Can you work these out from the model? Positions are in its coordinate system, mm. A direction names the side the tool comes from. Coordinates: 2 decimals unless noted, no trailing zeros. Order: outer loops, then holes, each group sorted by start corner. A loop starts at its lowest first (then second) coordinate and runs counter-clockwise, first axis right, second up. Notation, with made-up numbers: (66, 75.5) -> (91, 75.5) arc R8 ccw to (91, 83.5) -> close; hole circle Ø11 at (70.5, 45.25). An arc over 180 degrees is marked (long way). Answer in a Markdown table with one row per item. Add a question column.
1. Will these pins go through, and if not, where does the flat tip stop? pin 1 (0.9 mm diameter, centred on x = -39, z = -1, fed in from +Y); pin 2 (3 mm diameter, centred on y = -1, z = 6.5, fed in from +X); pin 3 (8 mm diameter, centred on x = -14.5, y = 0, fed in from +Z).
2. Imagine slicing it at B-B on x = 14. Write out the boundary of the cut face in (y, z), plus the area to 3 significant figures.
3. On a 3-axis mill with a long thin cutter (end or side, diameter ignored), from which of +Z, -Z, +X, -X, +Y, -Y can I reach the whole of each face in a straight line? I mean faces 5 (the face through (-0.7, 2.3, 0)), 6 (the face through (30.5, 0, 11)), 7 (the face through (-37, -9.6, -1.2)). Say none if no direction works.
4. Imagine slicing it at D-D on x = 46. Write out the boundary of the cut face in (y, z), plus the area to 3 significant figures.
5. Imagine slicing it at A-A on y = -8. Write out the boundary of the cut face in (x, z).
6. Imagine slicing it at C-C on z = 15. Write out the boundary of the cut face in (x, y).
7. If I drill on line 1 along Z through (x, y) = (34.5, 0.75); line 2 along Z through (x, y) = (34.5, -3.2); line 3 along Y through (x, z) = (14, 1.15), over which ranges is the centre line in solid material (lowest first)? Write a range as [from, to].
8. We'd pull the mould along Y, two halves only. Please class faces 1 (the face through (-38, -5, -1)), 2 (the face through (34, 0, 19)), 3 (the face through (-0.66, 1.05, 1.52)), 4 (the face through (35.4, -2, 14.1)): pulls with the +Y half, pulls with the -Y half, needs draft (parallel to the pull), parting line crosses it, or undercut.
from build123d import *

# Parameters (mm, degrees)
F0_W      = 105
F0_H      = 5
F1_DEPTH  = 3
F3_DEPTH  = 3.001
F4_R      = 3.5
F5_DEPTH  = 3.001
F6_DEPTH  = 3.001
F7_W      = 8
F7_H      = 10
F8_DEPTH  = 16
F9_R      = 1
F10_DEPTH = 10.001
F11_R     = 2
F12_DEPTH = 3
F13_W     = 5
F13_H     = 6
F14_DEPTH = 6
F15_R     = 1
F16_DEPTH = 93.001
F17_R     = 2
F18_DEPTH = 3


with BuildPart() as f1:
    # F0 (on Top) → F1 (new body)
    with BuildSketch(Plane.XY):
        with Locations((0, -2.5)):
            Rectangle(F0_W, F0_H)
        with Locations((0, 2.5)):
            Rectangle(F0_W, F0_H)
    extrude(amount=F1_DEPTH)

    # F2 (on face) → F3 (cut, through all)
    with BuildSketch(Plane.XY.offset(3)):
        with BuildLine():
            ThreePointArc((-44.5, 0), (-46, 1.5), (-47.5, 0))
            Line((-47.5, 0), (-44.5, 0))
        make_face()
        with BuildLine():
            ThreePointArc((47.5, 0), (46, 1.5), (44.5, 0))
            Line((44.5, 0), (47.5, 0))
        make_face()
        with BuildLine():
            Line((47.5, 0), (44.5, 0))
            ThreePointArc((44.5, 0), (46, -1.5), (47.5, 0))
        make_face()
        with BuildLine():
            Line((-44.5, 0), (-47.5, 0))
            ThreePointArc((-47.5, 0), (-46, -1.5), (-44.5, 0))
        make_face()
    extrude(amount=-F3_DEPTH, mode=Mode.SUBTRACT)

    # F4 (on face) → F5 (cut, through all)
    with BuildSketch(Plane.XY.offset(3)):
        with Locations((-4, 0)):
            Circle(F4_R)
        with Locations((14, 0)):
            Circle(F4_R)
    extrude(amount=-F5_DEPTH, mode=Mode.SUBTRACT)

    # F4 (on face) → F6 (cut, through all)
    with BuildSketch(Plane.XY.offset(3)):
        with Locations((-4, 0)):
            Circle(F4_R)
        with Locations((14, 0)):
            Circle(F4_R)
    extrude(amount=-F6_DEPTH, mode=Mode.SUBTRACT)

    # F7 (on face) → F8 (join)
    with BuildSketch(Plane.XY.offset(3)):
        with Locations((34.5, 0)):
            Rectangle(F7_W, F7_H)
    extrude(amount=F8_DEPTH)

    # F9 (on face) → F10 (cut, through all)
    with BuildSketch(Plane.XZ.offset(5)):
        with Locations((34.5, 15)):
            Circle(F9_R)
    extrude(amount=-F10_DEPTH, mode=Mode.SUBTRACT)

    # F11 (on face) → F12 (cut)
    with BuildSketch(Plane.XZ.offset(5)):
        with Locations((34.5, 15)):
            Circle(F11_R)
    extrude(amount=-F12_DEPTH, mode=Mode.SUBTRACT)

    # F13 (on face) → F14 (join)
    with BuildSketch(Plane.XY.offset(3)):
        with Locations((-38, -8)):
            Rectangle(F13_W, F13_H)
    extrude(amount=-F14_DEPTH)

    # F15 (on face) → F16 (cut, through all)
    with BuildSketch(Plane(origin=(-40.5, 0, 0), x_dir=(0, -1, 0), z_dir=(-1, 0, 0))):
        with Locations((8, 0)):
            Circle(F15_R)
    extrude(amount=-F16_DEPTH, mode=Mode.SUBTRACT)

    # F17 (on face) → F18 (cut)
    with BuildSketch(Plane.YZ.offset(-35.5)):
        with Locations((-8, 0)):
            Circle(F17_R)
    extrude(amount=-F18_DEPTH, mode=Mode.SUBTRACT)


solid = f1.part
Answers follow:
| question | item | result |
|---|---|---|
| 1 | pin 1 | stops at y = -5 |
| 1 | pin 2 | stops at x = 38.5 |
| 1 | pin 3 | stops at z = 3 |
| 2 | outline | (-5, 0) -> (-3.5, 0) -> (-3.5, 3) -> (-5, 3) -> close; (3.5, 0) -> (5, 0) -> (5, 3) -> (3.5, 3) -> close |
| 2 | area | 9.00 mm² |
| 3 | face 5 | -Z, +X, -X, +Y |
| 3 | face 6 | +Z, -X, +Y, -Y |
| 3 | face 7 | +X |
| 4 | outline | (-5, 0) -> (-1.5, 0) -> (-1.5, 3) -> (-5, 3) -> close; (1.5, 0) -> (5, 0) -> (5, 3) -> (1.5, 3) -> close |
| 4 | area | 21.0 mm² |
| 5 | outline | (-40.5, -3) -> (-35.5, -3) -> (-35.5, -2) -> (-38.5, -2) -> (-38.5, -1) -> (-40.5, -1) -> close; (-40.5, 1) -> (-38.5, 1) -> (-38.5, 2) -> (-35.5, 2) -> (-35.5, 3) -> (-40.5, 3) -> close |
| 6 | outline | (30.5, -5) -> (32.5, -5) -> (32.5, -2) -> (33.5, -2) -> (33.5, 5) -> (30.5, 5) -> close; (35.5, -2) -> (36.5, -2) -> (36.5, -5) -> (38.5, -5) -> (38.5, 5) -> (35.5, 5) -> close |
| 7 | line 1 | z = [0, 14], [16, 19] |
| 7 | line 2 | z = [0, 13], [17, 19] |
| 7 | line 3 | y = [-5, -3.5], [3.5, 5] |
| 8 | face 1 | pulls with the +Y half |
| 8 | face 2 | needs draft |
| 8 | face 3 | undercut |
| 8 | face 4 | pulls with the -Y half |
